CAD build for the part. Positions are in the model's coordinates, mm. Face numbers are marked on the shaded views. A direction names the side the tool comes from. Coordinates: 2 decimals unless noted, no trailing zeros. Loops run counter-clockwise (first coordinate to the right, second up) from the corner with the lowest first, then second, coordinate; pieces in that order, holes last.
1) Saw through at C-C, the plane z = 13.25. Give the number of separate pieces and of enclosed holes in the cut face, and give its area (3 significant figures).
2) Pin check, flat tips, straight feed: pin 1 Ø10 at (y, z) = (-0.5, 5) entering from -X; pin 2 Ø14 at (y, z) = (2.5, -7) entering from +X; pin 3 Ø1.5 at (x, z) = (14.5, -9) entering from -Y. Stop position of each tip, or through.
3) Two-plate mould, pull along X, no slides. Class the marked faces 1, 2 and 3: +X half, -X half, draft (parallel to the pull), parting line (faces both ways), or undercut.
4) Saw through at B-B, the plane x = 0. Write the cut outline in (y, z), and give its area (3 significant figures).
5) Which spindle directions (+Z, -Z, +X, -X, +Y, -Y) get a long thin tool onto all of the face, cutting with end or side? Do the marked faces 4, 5 and 6. Say none if no direction does.
6) Saw through at D-D, the plane y = -18. Write the cut outline in (x, z), and give its area (3 significant figures).
7) Saw through at A-A, the plane y = -31.5. Write the cut outline in (x, z).
8) Wall check: line 1 along Y through (x, z) = (31, 7); line 2 along Z through (x, y) = (0, -7); line 3 along X through (y, z) = (33.5, 11). Give the ranges that are in metal, low to high.
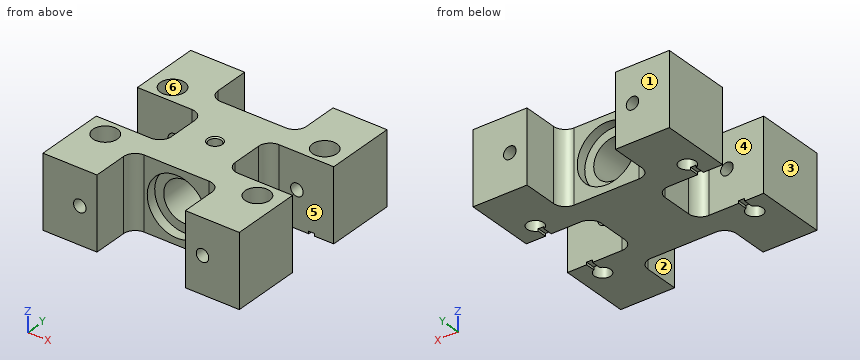
```python
from build123d import *

# Parameters (mm, degrees)
BOSS_EXTRUDE1_DEPTH                         = 14.75
CBORE_FOR_M6_HEX_HEAD_BOLT1_D               = 6.7
CBORE_FOR_M6_HEX_HEAD_BOLT1_CBORE_D         = 10
CBORE_FOR_M6_HEX_HEAD_BOLT1_CBORE_DEPTH     = 16
TAPPED_HOLE_FOR_10_32_HELICOIL1_D           = 5.1054
TAPPED_HOLE_FOR_10_32_HELICOIL1_DEPTH       = 11.9888
TAPPED_HOLE_FOR_10_32_HELICOIL1_CSINK_D     = 6.096
TAPPED_HOLE_FOR_10_32_HELICOIL1_CSINK_ANGLE = 90
TAPPED_HOLE_FOR_10_32_HELICOIL1_TIP         = 1.533816902
F_3_4_10_TAPPED_HOLE1_D                     = 16.66748
SKETCH11_R                                  = 12
CUT_EXTRUDE1_DEPTH                          = 4
SKETCH12_R                                  = 12
CUT_EXTRUDE2_DEPTH                          = 4
F_1_4_20_TAPPED_HOLE1_D                     = 5.1054
F_1_4_20_TAPPED_HOLE1_DEPTH                 = 28.5
F_1_4_20_TAPPED_HOLE2_D                     = 5.1054
F_1_4_20_TAPPED_HOLE2_DEPTH                 = 28.5
SKETCH20_W                                  = 2.36
SKETCH20_H                                  = 33.600070702
SKETCH20_H_2                                = 33.600816511
CUT_EXTRUDE3_DEPTH                          = 1


with BuildPart() as part:
    # Sketch1 → Boss-Extrude1 (new body, symmetric)
    with BuildSketch(Plane.XY):
        with BuildLine():
            Line((18, 39.5), (40, 39.5))
            Line((40, 39.5), (40, 11))
            Line((40, 11), (17.75, 11))
            ThreePointArc((17.75, 11), (14.391242789, 9.608757211), (13, 6.25))
            Line((13, 6.25), (13, -6.25))
            ThreePointArc((13, -6.25), (14.391242789, -9.608757211), (17.75, -11))
            Line((17.75, -11), (40, -11))
            Line((40, -11), (40, -39.5))
            Line((40, -39.5), (18, -39.5))
            Line((18, -39.5), (18, -25.25))
            ThreePointArc((18, -25.25), (16.608757211, -21.891242789), (13.25, -20.5))
            Line((13.25, -20.5), (-13.25, -20.5))
            ThreePointArc((-13.25, -20.5), (-16.608757211, -21.891242789), (-18, -25.25))
            Line((-18, -25.25), (-18, -39.5))
            Line((-18, -39.5), (-40, -39.5))
            Line((-40, -39.5), (-40, -11))
            Line((-40, -11), (-17.75, -11))
            ThreePointArc((-17.75, -11), (-14.391242789, -9.608757211), (-13, -6.25))
            Line((-13, -6.25), (-13, 6.25))
            ThreePointArc((-13, 6.25), (-14.391242789, 9.608757211), (-17.75, 11))
            Line((-17.75, 11), (-40, 11))
            Line((-40, 11), (-40, 39.5))
            Line((-40, 39.5), (-18, 39.5))
            Line((-18, 39.5), (-18, 25.25))
            ThreePointArc((-18, 25.25), (-16.608757211, 21.891242789), (-13.25, 20.5))
            Line((-13.25, 20.5), (13.25, 20.5))
            ThreePointArc((13.25, 20.5), (16.608757211, 21.891242789), (18, 25.25))
            Line((18, 25.25), (18, 39.5))
        make_face()
    extrude(amount=BOSS_EXTRUDE1_DEPTH, both=True)

    # CBORE for M6 Hex Head Bolt1 (through all)
    with Locations(Plane.XY.offset(14.75)):
        with Locations((31, 18), (-31, 18), (-31, -18), (31, -18)):
            CounterBoreHole(CBORE_FOR_M6_HEX_HEAD_BOLT1_D / 2, CBORE_FOR_M6_HEX_HEAD_BOLT1_CBORE_D / 2, CBORE_FOR_M6_HEX_HEAD_BOLT1_CBORE_DEPTH)

    # Tapped Hole for #10-32 Helicoil1
    with Locations(Plane.XY.offset(14.75)):
        with Locations((0, 0)):
            CounterSinkHole(TAPPED_HOLE_FOR_10_32_HELICOIL1_D / 2, TAPPED_HOLE_FOR_10_32_HELICOIL1_CSINK_D / 2, depth=TAPPED_HOLE_FOR_10_32_HELICOIL1_DEPTH, counter_sink_angle=TAPPED_HOLE_FOR_10_32_HELICOIL1_CSINK_ANGLE)
            with Locations((0, 0, -(TAPPED_HOLE_FOR_10_32_HELICOIL1_DEPTH + TAPPED_HOLE_FOR_10_32_HELICOIL1_TIP / 2))):  # 118° drill point
                Cone(0, TAPPED_HOLE_FOR_10_32_HELICOIL1_D / 2, TAPPED_HOLE_FOR_10_32_HELICOIL1_TIP, mode=Mode.SUBTRACT)

    # 3/4-10 Tapped Hole1 (through all)
    with Locations(Plane(origin=(0, 20.5, 0), x_dir=(-1, 0, 0), z_dir=(0, 1, 0))):
        with Locations((0, 0)):
            Hole(F_3_4_10_TAPPED_HOLE1_D / 2)

    # Sketch11 → Cut-Extrude1 (cut)
    with BuildSketch(Plane(origin=(0, 20.5, 0), x_dir=(1, 0, 0), z_dir=(0, 1, 0))):
        with Locations(Location((0, 0, 0), (0, 0, 270))):  # turned: the seam where the file's is
            Circle(SKETCH11_R)
    extrude(amount=-CUT_EXTRUDE1_DEPTH, mode=Mode.SUBTRACT)

    # Sketch12 → Cut-Extrude2 (cut)
    with BuildSketch(Plane.XZ.offset(20.5)):
        with Locations(Location((0, 0, 0), (0, 0, 90))):  # turned: the seam where the file's is
            Circle(SKETCH12_R)
    extrude(amount=-CUT_EXTRUDE2_DEPTH, mode=Mode.SUBTRACT)

    # 1/4-20 Tapped Hole1
    with Locations(Plane(origin=(0, 39.5, 0), x_dir=(-1, 0, 0), z_dir=(0, 1, 0))):
        with Locations((-25, 0.25), (25, 0.25)):
            Hole(F_1_4_20_TAPPED_HOLE1_D / 2, depth=F_1_4_20_TAPPED_HOLE1_DEPTH)

    # 1/4-20 Tapped Hole2
    with Locations(Plane.XZ.offset(39.5)):
        with Locations((25, 0.25), (-25, 0.25)):
            Hole(F_1_4_20_TAPPED_HOLE2_D / 2, depth=F_1_4_20_TAPPED_HOLE2_DEPTH)

    # Sketch20 → Cut-Extrude3 (cut)
    with BuildSketch(Plane(origin=(0, 0, -14.75), x_dir=(-1, 0, 0), z_dir=(0, 0, -1))):
        with Locations((31, -0.882383927)):
            Rectangle(SKETCH20_W, SKETCH20_H)
        with Locations((-31, -0.882756832)):
            Rectangle(SKETCH20_W, SKETCH20_H_2)
    extrude(amount=-CUT_EXTRUDE3_DEPTH, mode=Mode.SUBTRACT)


solid = part.part
```
Data:
1. separate pieces: 1
1. enclosed holes: 5
1. area: 3,470 mm2
2. pin 1: stops at x = -13
2. pin 2: stops at x = 14.29
2. pin 3: stops at y = -20.94
3. face 1: draft
3. face 2: undercut
3. face 3: -X half
4. outline: (-20.5, -14.75) - (20.5, -14.75) - (20.5, -12) - (16.5, -12) - (16.5, -8.33) - (-16.5, -8.33) - (-16.5, -12) - (-20.5, -12) - close; (-20.5, 12) - (-16.5, 12) - (-16.5, 8.33) - (-2.55, 8.33) - (-2.55, 14.25) - (-3.05, 14.75) - (-20.5, 14.75) - close; (2.55, 8.33) - (16.5, 8.33) - (16.5, 12) - (20.5, 12) - (20.5, 14.75) - (3.05, 14.75) - (2.55, 14.25) - close
4. area: 434 mm2
5. face 4: +Z, -Z, -X
5. face 5: +Z, -Z, +X
5. face 6: +Z
6. outline: (-40, -14.75) - (-34.35, -14.75) - (-34.35, -1.25) - (-36, -1.25) - (-36, 14.75) - (-40, 14.75) - close; (-27.65, -14.75) - (27.65, -14.75) - (27.65, -1.25) - (27.07, -1.25) arc R2.55 cw (long way) to (26, 2.6) - (26, 14.75) - (-26, 14.75) - (-26, 2.6) arc R2.55 cw (long way) to (-27.07, -1.25) - (-27.65, -1.25) - close; (34.35, -14.75) - (40, -14.75) - (40, 14.75) - (36, 14.75) - (36, -1.25) - (34.35, -1.25) - close; hole circle Ø24 at (0, 0)
6. area: 1,380 mm2
7. outline: (-40, -14.75) - (-18, -14.75) - (-18, 14.75) - (-40, 14.75) - close; (18, -14.75) - (40, -14.75) - (40, 14.75) - (18, 14.75) - close; hole circle Ø5.11 at (-25, 0.25); hole circle Ø5.11 at (25, 0.25)
8. line 1: y = -39.5 to -23, -13 to -11, 11 to 13, 23 to 39.5
8. line 2: z = -14.75 to -8.33, 8.33 to 14.75
8. line 3: x = -40 to -18, 18 to 40
